Model file for the job. Use its own axes, mm. A direction names the side the tool comes from. Round coordinates to 2 decimals unless told otherwise and drop trailing zeros. Loops run counter-clockwise (first coordinate to the right, second up) from the corner with the lowest first, then second, coordinate; pieces in that order, holes last. Notation, with made-up numbers: M -2.75,-39 L 23.25,-39 A16 cw 23.25,-9 Z; hole C -37.75,39 d8. An arc over 180 degrees is marked long. Use a Markdown table: item, result. Add a question column.
Item 1: Two-plate mould, pull along Z, no slides. Class faces 4 (the cylindrical face through (100.503, 1.565, 0.862)), 5 (the cylindrical face through (110.735, 1.565, 12.116)), 6 (the flat face through (38, 0, 15)): +Z half, -Z half, draft (parallel to the pull), parting line (faces both ways), or undercut.
Item 2: Pin check, flat tips, straight feed: P1, Ø3.5, axis at x = 98.425, z = 0, coming from the +Y side; P2, Ø1.6, axis at x = -4.5, y = 2, coming from the +Z side (3 decimals); P3, Ø1, axis at y = 2.5, z = 49, coming from the -X side. Stop position of each tip, or through.
Item 3: Saw through at B-B on y = 2.6. Give the number of separate pieces and of enclosed holes in the cut face, then the cut area to 3 significant figures.
Item 4: Wall check: L1, parallel to Z at x = 50.8, y = 0.85 (3 decimals); L2, parallel to X at y = 1.55, z = 41.5; L3, parallel to Z at x = 7, y = 1.4 (3 decimals). Give the ranges that are in metal, low to high. Write a range as from..to.
Item 5: Saw through at A-A on z = 0. Write the cut outline in (x, y) (3 decimals).
Item 6: Tool access for faces 1 (the flat face through (83, 2, 15.875)), 2 (the flat face through (0, 2, 41)), 3 (the cylindrical face through (43.69, 1.57, 30)): list every direction of +Z, -Z, +X, -X, +Y, -Y with a clear straight run to the whole face (end or side of a thin tool).
Item 7: Saw through at C-C on z = 54. Write the cut outline in (x, y) (3 decimals), then the cut area to 3 significant figures.
```python
from build123d import *

# Parameters (mm, degrees)
SKETCH1_R           = 3
SKETCH1_R_2         = 2.25
BOSS_EXTRUDE1_DEPTH = 3.175


with BuildPart() as part:
    # Sketch1 → Boss-Extrude1 (new body)
    with BuildSketch(Plane(origin=(0, 0, 0), x_dir=(1, 0, 0), z_dir=(0, 1, 0))):
        with BuildLine():
            Line((-12.7, -15.875), (-12.7, 15.875))
            Line((-12.7, 15.875), (101.8, 15.875))
            ThreePointArc((101.8, 15.875), (110.638834765, 12.213834765), (114.3, 3.375))
            Line((114.3, 3.375), (114.3, -3.375))
            ThreePointArc((114.3, -3.375), (110.638834765, -12.213834765), (101.8, -15.875))
            Line((101.8, -15.875), (63.5, -15.875))
            ThreePointArc((63.5, -15.875), (40.28137649, -51.591436626), (0, -65.454301807))
            Line((0, -65.454301807), (0, -15.875))
            Line((0, -15.875), (-12.7, -15.875))
        make_face()
        Circle(SKETCH1_R, mode=Mode.SUBTRACT)
        with Locations((98.425, 0)):
            Circle(SKETCH1_R_2, mode=Mode.SUBTRACT)
        with Locations((50.8, 0)):
            Circle(SKETCH1_R_2, mode=Mode.SUBTRACT)
        with Locations((49.750497609, -10.272681618)):
            Circle(SKETCH1_R_2, mode=Mode.SUBTRACT)
        with Locations((46.645354818, -20.120906389)):
            Circle(SKETCH1_R_2, mode=Mode.SUBTRACT)
        with Locations((41.612872995, -29.137755595)):
            Circle(SKETCH1_R_2, mode=Mode.SUBTRACT)
        with Locations((34.860989216, -36.950662117)):
            Circle(SKETCH1_R_2, mode=Mode.SUBTRACT)
        with Locations((26.66868451, -43.236804536)):
            Circle(SKETCH1_R_2, mode=Mode.SUBTRACT)
        with Locations((17.374456649, -47.736445785)):
            Circle(SKETCH1_R_2, mode=Mode.SUBTRACT)
        with Locations((7.362333757, -50.263665223)):
            Circle(SKETCH1_R_2, mode=Mode.SUBTRACT)
        with Locations((38.1, 0)):
            Circle(SKETCH1_R_2, mode=Mode.SUBTRACT)
    extrude(amount=BOSS_EXTRUDE1_DEPTH)


solid = part.part
```
Entries:
| question | item | result |
|---|---|---|
| 1 | face 4 | undercut |
| 1 | face 5 | +Z half |
| 1 | face 6 | draft |
| 2 | P1 | through |
| 2 | P2 | z = 15.875 |
| 2 | P3 | x = 0 |
| 3 | separate pieces | 1 |
| 3 | enclosed holes | 11 |
| 3 | area | 6,110 mm2 |
| 4 | L1 | -15.875..-2.25, 2.25..8.282, 12.263..41.275 |
| 4 | L2 | 0..25.24, 28.1..50.62 |
| 4 | L3 | -15.875..48.043, 52.484..65.079 |
| 5 | outline | M -12.7,0 L -3,0 L -3,3.175 L -12.7,3.175 Z; M 3,0 L 35.85,0 L 35.85,3.175 L 3,3.175 Z; M 40.35,0 L 48.55,0 L 48.55,3.175 L 40.35,3.175 Z; M 53.05,0 L 96.175,0 L 96.175,3.175 L 53.05,3.175 Z; M 100.675,0 L 114.3,0 L 114.3,3.175 L 100.675,3.175 Z |
| 6 | face 1 | +Z, +X, +Y, -Y |
| 6 | face 2 | +Z, -X, +Y, -Y |
| 6 | face 3 | +Y, -Y |
| 7 | outline | M 0,0 L 36.99,0 L 36.99,3.175 L 0,3.175 Z |
| 7 | area | 117 mm2 |
